Here's how the part is built. I have some questions about the finished solid (model axes, mm). Round coordinates to 2 decimals unless told otherwise and drop trailing zeros. Loops run counter-clockwise (first coordinate to the right, second up) from the corner with the lowest first, then second, coordinate; pieces in that order, holes last. Notation, with made-up numbers: (18, -25) - (74, -25) arc R24 cw to (74, 10) - close; hole circle Ø10 at (-10, 37.5). An arc over 180 degrees is marked (long way). Answer as a JSON object with one key per item and string values. Group by question number.
1) I want a section at D-D, the plane y = 36.5. Please give me the cut outline in (x, z), then the cut area to 3 significant figures.
2) I want a section at B-B, the plane z = 6.35. Please give me the cut outline in (x, y), then the cut area to 3 significant figures.
3) I want a section at A-A, the plane y = 5. Please give me the cut outline in (x, z).
4) If I drill on line 1 along X through (y, z) = (75, 3.5); line 2 along X through (y, z) = (5, 7); line 3 along Y through (x, z) = (8.5, 2.5), over which ranges is the centre line in solid material (lowest first)? Write a range as [from, to].
5) Will this pin go through, and if not, where does the flat tip stop? P1, Ø2.5, axis at x = 6.35, y = 75, coming from the +Z side.
6) I want a section at C-C, the plane x = 6.35. Please give me the cut outline in (y, z).
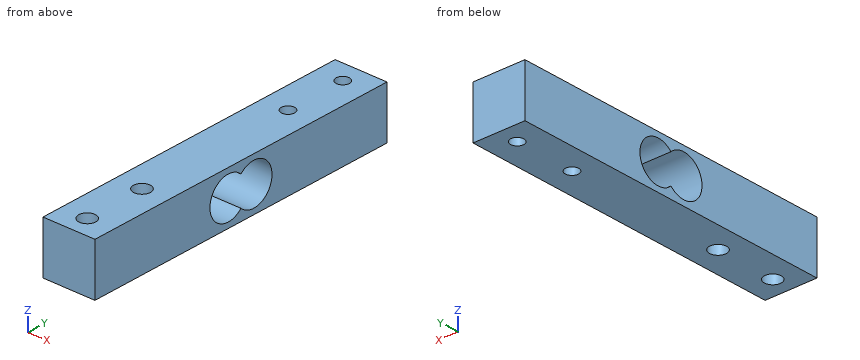
Autodesk Inventor part; units mm, degrees
ref_plane "YZ Plane" through (0, 0, 0) normal (1, 0, 0) x (0, 1, 0)
ref_plane "XZ Plane" through (0, 0, 0) normal (0, 1, 0) x (-1, 0, 0)
ref_plane "XY Plane" through (0, 0, 0) normal (0, 0, 1) x (1, 0, 0)
sketch "Skizze1" plane through (0, 0, 0) normal (0, 0, 1) x (1, 0, 0)
  line L0 (0, 0) -> (12.7, 0)
  line L1 (12.7, 0) -> (12.7, 80)
  line L2 (12.7, 80) -> (0, 80)
  line L3 (0, 80) -> (0, 0)
  dimension "d0" = 12.7
  dimension "d1" = 80
extrude "Extrusion1" add sketch "Skizze1" along normal blind 12.7
sketch "Skizze2" plane through (0, 0, 12.7) normal (0, 0, 1) x (1, 0, 0)
  line L0 (0, 0) -> (12.7, 0)
  line L1 (6.35, 0) -> (5, 0)
  line L2 (5, 0) -> (5, 5)
  line L3 (5, 5) -> (6.35, 5)
  line L4 (6.35, 5) -> (6.35, 0)
  line L5 (6.35, 5) -> (2, 5)
  line L6 (2, 5) -> (2, 20)
  line L7 (2, 20) -> (6.35, 20)
  line L8 (6.35, 20) -> (6.35, 5)
  dimension "d4" = 5
  dimension "d5" = 15
hole "Bohrung1" at (6.35, 5, 12.7) at (6.35, 20, 12.7) direction (0, 0, -1) diameter 4.134 end through all
sketch "Skizze3" plane through (0, 0, 12.7) normal (0, 0, 1) x (1, 0, 0)
  line L0 (12.7, 80) -> (0, 80)
  line L1 (6.35, 80) -> (4, 80)
  line L2 (4, 80) -> (4, 75)
  line L3 (4, 75) -> (6.35, 75)
  line L4 (6.35, 75) -> (6.35, 80)
  line L5 (6.35, 75) -> (4, 75)
  line L6 (4, 75) -> (4, 60)
  line L7 (4, 60) -> (6.35, 60)
  line L8 (6.35, 60) -> (6.35, 75)
  point P0 (0, 0)
  dimension "d13" = 5
  dimension "d14" = 15
hole "Bohrung2" at (6.35, 60, 12.7) at (6.35, 75, 12.7) direction (0, 0, -1) diameter 3.242 end through all
sketch "Skizze4" plane through (12.7, 0, 0) normal (1, 0, 0) x (0, 0, -1)
  line L0 (0, 0) -> (-12.7, 0)
  line L1 (-12.7, 0) -> (-12.7, 80)
  line L2 (-6.35, 0) -> (-12.7, 0)
  line L3 (-12.7, 0) -> (-12.7, 40)
  line L4 (-12.7, 40) -> (-6.35, 40)
  line L5 (-6.35, 40) -> (-6.35, 0)
  line L6 (-6.35, 36.5) -> (-6.35, 43.5)
  line L7 (-6.35, 43.5) -> (-6.35, 36.5)
  circle A0 centre (-6.35, 36.5) radius 5
  circle A1 centre (-6.35, 43.5) radius 5
  point P0 (-6.35, 40)
  dimension "d22" = 7
  dimension "d23" = 10
  dimension "d24" = 10
extrude "Extrusion2" cut sketch "Skizze4" against normal through all contours A0 A1 L5 | L5 A1 A0 | A0 L6 L4 | A1 A0 | L4 L5 A1 | L5 L6 A0 A1
equation "\"d24\" = d23"
properties part number "LoadCell"
Outcome:
{
 "1": {"outline": "(0, 0) - (12.7, 0) - (12.7, 1.35) - (0, 1.35) - close; (0, 11.35) - (12.7, 11.35) - (12.7, 12.7) - (0, 12.7) - close", "area": "34.3 mm^2"},
 "2": {"outline": "(0, 0) - (12.7, 0) - (12.7, 31.5) - (0, 31.5) - close; (0, 48.5) - (12.7, 48.5) - (12.7, 80) - (0, 80) - close; hole circle Ø4.13 at (6.35, 5); hole circle Ø4.13 at (6.35, 20); hole circle Ø3.24 at (6.35, 60); hole circle Ø3.24 at (6.35, 75)", "area": "757 mm^2"},
 "3": {"outline": "(0, 0) - (4.28, 0) - (4.28, 12.7) - (0, 12.7) - close; (8.42, 0) - (12.7, 0) - (12.7, 12.7) - (8.42, 12.7) - close"},
 "4": {"line 1": "[0, 4.73], [7.97, 12.7]", "line 2": "[0, 4.28], [8.42, 12.7]", "line 3": "[0, 33.31], [39.69, 40.31], [46.69, 80]"},
 "5": {"P1": "through"},
 "6": {"outline": "(0, 0) - (2.93, 0) - (2.93, 12.7) - (0, 12.7) - close; (7.07, 0) - (17.93, 0) - (17.93, 12.7) - (7.07, 12.7) - close; (22.07, 0) - (58.38, 0) - (58.38, 12.7) - (22.07, 12.7) - close; (61.62, 0) - (73.38, 0) - (73.38, 12.7) - (61.62, 12.7) - close; (76.62, 0) - (80, 0) - (80, 12.7) - (76.62, 12.7) - close; hole (40, 2.78) arc R5 ccw (long way) to (40, 9.92) arc R5 ccw (long way) to start"}
}
